Build history of the part. All positions in model axes, mm. A direction names the side the tool comes from. Give positions to 0.01 mm unless a question says otherwise; leave off trailing zeros. Order: outer loops, then holes, each group sorted by start corner. A loop starts at its lowest first (then second) coordinate and runs counter-clockwise, first axis right, second up. Notation, with made-up numbers: M 20.25,59 L 36.25,59 A10 cw 36.25,76 Z; hole C 19,49.25 d8. An arc over 180 degrees is marked long. Answer as CSV lines item,"result".
from build123d import *

# Parameters (mm, degrees)
F1_DEPTH = 100
F4_DEPTH = 17.5
F5_DEPTH = 2.5


with BuildPart() as f1:
    # F0 (on Top) → F1 (new body)
    with BuildSketch(Plane.XY):
        with BuildLine():
            ThreePointArc((28.5209304486, -23.5702466331), (12.2876501905, -3.9924995673), (36.9281607922, 2.3045477884))
            ThreePointArc((36.9281607922, 2.3045477884), (34.9662176525, 12.0980834464), (30.4561960313, 21.0100005546))
            ThreePointArc((30.4561960313, 21.0100005546), (8.8261833484, 12.1481991875), (10.5702157772, 35.4580109203))
            ThreePointArc((10.5702157772, 35.4580109203), (-0.6938621952, 36.9934934178), (-11.8924377724, 35.0366939626))
            ThreePointArc((-11.8924377724, 35.0366939626), (-6.8453800934, 30.4634762693), (-4.9749320578, 23.9145423537))
            ThreePointArc((-4.9749320578, 23.9145423537), (-16.4840155326, 11.5465890976), (-29.6469107264, 22.1373142992))
            ThreePointArc((-29.6469107264, 22.1373142992), (-35.4260679906, 10.6767835385), (-36.9421307963, -2.0685676756))
            ThreePointArc((-36.9421307963, -2.0685676756), (-25.064120667, 0.6380392173), (-18.2026853687, -9.4284175154))
            ThreePointArc((-18.2026853687, -9.4284175154), (-22.1469156931, -17.7804681058), (-31.1026851957, -20.0405332668))
            ThreePointArc((-31.1026851957, -20.0405332668), (-23.7959360481, -28.3329036209), (-14.3659429831, -34.0972093023))
            ThreePointArc((-14.3659429831, -34.0972093023), (-3.3658654806, -12.0826767357), (15.8, -27.52))
            ThreePointArc((15.8, -27.52), (15.4373232643, -30.8858654806), (14.3659429831, -34.0972093023))
            ThreePointArc((14.3659429831, -34.0972093023), (22.0799731419, -29.6896410563), (28.5209304486, -23.5702466331))
        make_face()
    extrude(amount=F1_DEPTH)

    # F3 (on offset) → F4 (join)
    with BuildSketch(Plane.XY.offset(100)):
        with BuildLine():
            ThreePointArc((0, -5), (3.5355339059, -3.5355339059), (5, 0))
            ThreePointArc((5, 0), (0, 5), (-5, 0))
            Line((-5, 0), (0, -5))
        make_face()
    extrude(amount=F4_DEPTH)

    # F3 (on offset) → F5 (join)
    with BuildSketch(Plane.XY.offset(100)):
        with BuildLine():
            Line((0, -5), (-5, 0))
            ThreePointArc((-5, 0), (-3.5355339059, -3.5355339059), (0, -5))
        make_face()
    extrude(amount=F5_DEPTH)


solid = f1.part
Item 1: Pull direction X, two halves, no side cores. Call faces 1 (the flat face through (0, 0, 117.5)), 2 (the cylindrical face through (-23.915, -28.233, 49.3)), 3 (the cylindrical face through (-0.442, -11.726, 49.3)), 4 (the cylindrical face through (9.15, 11.92, 49.3)): released by +X, released by -X, zero draft, split by the parting line, or undercut.
Geometry says:
face 1,"zero draft"
face 2,"released by -X"
face 3,"undercut"
face 4,"undercut"
Item 2: Band-saw the part on A-A (y = -27.52). Give the cut face in (x, z).
Geometry says:
outline,"M -24.73,0 L -15.8,0 L -15.8,100 L -24.73,100 Z; M 15.8,0 L 24.73,0 L 24.73,100 L 15.8,100 Z"
Item 3: 3-axis set-ups, long thin cutter, end or side, ignore diameter. For faces 5 (the flat face through (-3, -2, 110)), 6 (the cylindrical face through (-0.534, 36.996, 49.3)): which of +Z, -Z, +X, -X, +Y, -Y reach the whole face in a straight line?
Geometry says:
face 5,"+Z, -X, -Y"
face 6,"+Z, -Z, +Y"
Item 4: Band-saw the part on B-B (z = 85). Give the cut face in (x, y) (3 decimals).
Geometry says:
outline,"M -36.942,-2.069 A10.815 cw long -31.103,-20.041 A37 ccw -14.366,-34.097 A15.8 cw long 14.366,-34.097 A37 ccw 28.521,-23.57 A15.05 cw long 36.928,2.305 A37 ccw 30.456,21.01 A13.74 cw long 10.57,35.458 A37 ccw -11.892,35.037 A12.4 cw long -29.647,22.137 A37 ccw Z"
Item 5: Drop flat-ended pins along their axis: pin 1 (12 mm diameter, centred on y = 19.5, z = 83.5, fed in from +X); pin 2 (8 mm diameter, centred on x = -19.5, z = 20.5, fed in from -Y); pin 3 (4 mm diameter, centred on x = -22, z = 54, fed in from +Y). Give the stop position or say it passes through.
Geometry says:
pin 1,"stops at x = 34.45"
pin 2,"stops at y = -33.6"
pin 3,"stops at y = 13.43"
Item 6: Band-saw the part on C-C (x = 22). Give the cut face in (y, z), and give its area (3 significant figures).
Geometry says:
outline,"M -29.75,0 L -22.97,0 L -22.97,100 L -29.75,100 Z; M 5.69,0 L 10.5,0 L 10.5,100 L 5.69,100 Z"
area,"1,160 mm2"
Item 7: Probe line 1 along X through (y, z) = (20, 13.5); line 2 along X through (y, z) = (18, 23); line 3 along Z through (x, y) = (3, 32.5). List the from-to ranges inside material, lowest first. Write a range as from..to.
Geometry says:
line 1,"x = -31.13..-29.14, -5.61..3.56, 30.25..31.13"
line 2,"x = -32.33..-28.27, -6.48..4.21, 29.59..32.33"
line 3,"z = 0..100"
